from build123d import *

# Parameters (mm, degrees)
PAD_DEPTH = 6


with BuildPart() as part:
    # Sketch → Pad (new body)
    with BuildSketch(Plane.XY):
        with BuildLine():
            Line((0, 0), (113, 0))
            Line((113, 0), (113, 12))
            Line((113, 12), (107, 12))
            Line((107, 12), (107, 24))
            Line((107, 24), (113, 24))
            Line((113, 24), (113, 35))
            ThreePointArc((113, 35), (101.284271, 63.284271), (73, 75))
            Line((73, 75), (0, 75))
            Line((-73, 75), (0, 75))
            ThreePointArc((-73, 75), (-101.284271, 63.284271), (-113, 35))
            Line((-113, 24), (-113, 35))
            Line((-107, 24), (-113, 24))
            Line((-107, 12), (-107, 24))
            Line((-113, 12), (-107, 12))
            Line((-113, 0), (-113, 12))
            Line((0, 0), (-113, 0))
        make_face()
    extrude(amount=PAD_DEPTH)


solid = part.part
Input: part model. Units: mm. Frame: model coordinates. A direction names the side the tool comes from. Round coordinates to 2 decimals unless told otherwise and drop trailing zeros. Order: outer loops, then holes, each group sorted by start corner. A loop starts at its lowest first (then second) coordinate and runs counter-clockwise, first axis right, second up. Notation, with made-up numbers: (7.5, 19.5) - (58.5, 19.5) arc R13 ccw to (58.5, 25.5) - close; hole circle Ø2 at (64.25, -33.5). An arc over 180 degrees is marked (long way). Answer as a JSON object with one key per item and string values. Group by question number.
(1) Cut plane A-A (z = 1.6). Return loops of the section in (x, y).
(2) Cut plane C-C (y = 70). Return loops of the section in (x, z), then the cut area to 3 significant figures.
(3) Material intervals for probe 1 along X at (y, z) = (15, 0.35); probe 2 along Y at (x, z) = (85, 1.05); probe 3 along Y at (x, z) = (82, 3.8), sorted ascending. Write a range as from..to.
(4) Cut plane B-B (x = 97). Return loops of the section in (y, z).
(5) Reachability of faces 1 (the face through (-2, 38, 6)), 2 (the face through (110, 12, 3)), 3 (the face through (-110, 12, 3)) from +Z, -Z, +X, -X, +Y, -Y: full face, straight path, thin tool, end or side. Return the list, or none.
(6) Pin query (flat end, axial travel): P1, Ø3, axis at x = -111.5, z = 2, coming from the +Y side; P2, Ø1, axis at y = 64.5, z = 5.5, coming from the -X side; P3, Ø1.8, axis at y = 20.5, z = 3.5, coming from the +X side. Return the tip coordinate at first contact, or that it passes through.
(7) Draft query along Y for faces 4 (the face through (113, 6, 3)), 5 (the face through (-107, 18, 3)), 6 (the face through (101.594, 62.972, 2.958)), 7 (the face through (-2, 0, 3)). Return one class per face: released by +Y, released by -Y, zero draft, split by the parting line, or undercut.
Here are the results:
{
 "1": {"outline": "(-113, 0) - (113, 0) - (113, 12) - (107, 12) - (107, 24) - (113, 24) - (113, 35) arc R40 ccw to (73, 75) - (-73, 75) arc R40 ccw to (-113, 35) - (-113, 24) - (-107, 24) - (-107, 12) - (-113, 12) - close"},
 "2": {"outline": "(-92.36, 0) - (92.36, 0) - (92.36, 6) - (-92.36, 6) - close", "area": "1,110 mm^2"},
 "3": {"probe 1": "x = -107..107", "probe 2": "y = 0..73.16", "probe 3": "y = 0..73.97"},
 "4": {"outline": "(0, 0) - (67, 0) - (67, 6) - (0, 6) - close"},
 "5": {"face 1": "+Z, +X, -X, +Y, -Y", "face 2": "+Z, -Z, +X", "face 3": "+Z, -Z, -X"},
 "6": {"P1": "stops at y = 50.2", "P2": "stops at x = -100.55", "P3": "stops at x = 107"},
 "7": {"face 4": "zero draft", "face 5": "undercut", "face 6": "released by +Y", "face 7": "released by -Y"}
}
